Study the drawing (mm; zero at the part's minimum x, y, z) and answer. Round coordinates to 2 decimals unless told otherwise and drop trailing zeros. Order: outer loops, then holes, each group sorted by start corner. A loop starts at its lowest first (then second) coordinate and runs counter-clockwise, first axis right, second up. Notation, with made-up numbers: (63, 11.25) - (91, 11.25) arc R16 ccw to (91, 17.25) - close; hole circle Ø8 at (16.25, 52.5). An arc over 180 degrees is marked (long way). Use one line per item in the form item = value. Start each with the question number.
Q1. The part is cut by section B-B on x = 50. Determine the outline of the cut face in (y, z) (1 decimal).
Q2. Given P1, Ø1, axis at y = 52, z = 1, coming from the +X side (1 decimal), flat-ended and moving along its own axis, determine where the tip first touches the part or whether it passes through.
Q3. The part is cut by section A-A on y = 26.5. Determine the outline of the cut face in (x, z) (1 decimal).
Q4. Find the intervals of material crossed by line 1 (X direction, y = 28, z = 1.9) (1 decimal); line 2 (X direction, y = 38, z = 1.2); line 3 (Y direction, x = 20.5, z = 0.4), in increasing order. Write a range as [from, to].
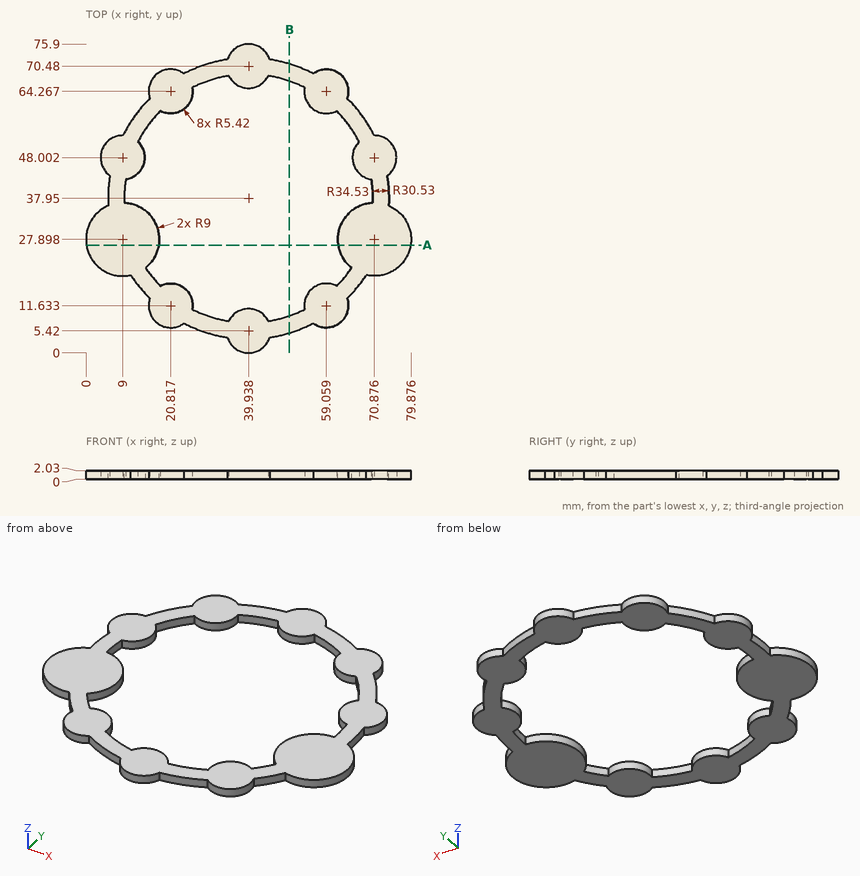
Found:
q1.outline = (4.9, 0) - (9.1, 0) - (9.1, 2) - (4.9, 2) - close; (66.8, 0) - (71, 0) - (71, 2) - (66.8, 2) - close
q2.P1 = 75
q3.outline = (0.1, 0) - (17.9, 0) - (17.9, 2) - (0.1, 2) - close; (62, 0) - (79.8, 0) - (79.8, 2) - (62, 2) - close
q4.line_1 = [0, 18], [61.9, 79.9]
q4.line_2 = [5.41, 9.41], [70.47, 74.47]
q4.line_3 = [6.22, 17.04], [58.86, 69.68]
